from build123d import *

# Parameters (mm, degrees)
F1_R     = 10
F2_DEPTH = 9.2
F3_R     = 37.5
F4_DEPTH = 29.6
F5_R     = 30.5
F6_DEPTH = 25.8
F7_R     = 26.905
F8_DEPTH = 0.35


# Not quite as in the source:
# - a fillet or chamfer that OpenCascade refuses, or shapes differently, is made with other operations: its cross-section is extruded or revolved along the edge and cut away or added


with BuildPart() as f2:
    # F1 (on Top) → F2 (new body)
    with BuildSketch(Plane.XY):
        Circle(F1_R)
    extrude(amount=F2_DEPTH)

    # F3 (on face) → F4 (join)
    with BuildSketch(Plane.XY.offset(9.2)):
        Circle(F3_R)
    extrude(amount=F4_DEPTH)

    # F5 (on face) → F6 (join)
    with BuildSketch(Plane.XY.offset(38.8)):
        Circle(F5_R)
    extrude(amount=F6_DEPTH)

    # F7 (on face) → F8 (cut)
    with BuildSketch(Plane.XY.offset(64.6)):
        Circle(F7_R)
    extrude(amount=-F8_DEPTH, mode=Mode.SUBTRACT)

    # F10: chamfer of 0.5 on 2 edges, made by hand


with BuildPart() as f10_tool2:
    # F10_s3 → F10_t4 (revolve)
    with BuildSketch(Plane.XZ):
        Polygon((27.405, 64.6), (26.905, 64.1), (26.905, 64.6), align=None)
    revolve(axis=Axis((0, 0, 64.6), (0, 0, 1)))

    split(bisect_by=Plane.XY.offset(64.25), keep=Keep.TOP)


with BuildPart() as f2_1:
    add(f2.part)

    # F10_t1: cut F10_tool2
    add(f10_tool2.part, mode=Mode.SUBTRACT)

    # F10_s6 → F10_t7 (revolve, cut)
    with BuildSketch(Plane.XZ):
        Polygon((10, 0.5), (9.5, 0), (10, 0), align=None)
    revolve(axis=Axis((0, 0, 0), (0, 0, 1)), mode=Mode.SUBTRACT)

    # F11 (on Front) → F12 (revolve)
    with BuildSketch(Plane.XZ):
        Polygon((0, 64.25), (0, 74.65), (-19.25, 74.65), (-19.975, 68.05), (-19.975, 64.25), align=None)
    revolve(axis=Axis((0, 0, 44.8884957004), (0, 0, -1)))


solid = f2_1.part
Can you work these out from the model? Positions are in its coordinate system, mm. A direction names the side the tool comes from. Give positions to 0.01 mm unless a question says otherwise; leave off trailing zeros. Order: outer loops, then holes, each group sorted by start corner. A loop starts at its lowest first (then second) coordinate and runs counter-clockwise, first axis right, second up. Notation, with made-up numbers: M -23,8.25 L 12,8.25 A26 cw 12,44.25 Z; hole C -6.75,-2.75 d3. An arc over 180 degrees is marked long. Use one line per item in the form item = value.
Item 1: If we section it at D-D, the plane x = -29: Write out the boundary of the cut face in (y, z).
Values follow:
outline = M -23.77,9.2 L 23.77,9.2 L 23.77,38.8 L 9.45,38.8 L 9.45,64.6 L -9.45,64.6 L -9.45,38.8 L -23.77,38.8 Z
Item 2: If I drill on line 1 along Z through (x, y) = (-23, 5); line 2 along Y through (x, z) = (1, 12); line 3 along Z through (x, y) = (-33, -12.5), over which ranges is the centre line in solid material (lowest first)? Write a range as [from, to].
Values follow:
line_1 = [9.2, 64.25]
line_2 = [-37.49, 37.49]
line_3 = [9.2, 38.8]
Item 3: If we section it at A-A, the plane y = 0: Write out the boundary of the cut face in (x, z) (3 decimals), and give its area (3 significant figures).
Values follow:
outline = M -37.5,9.2 L -10,9.2 L -10,0.5 L -9.5,0 L 9.5,0 L 10,0.5 L 10,9.2 L 37.5,9.2 L 37.5,38.8 L 30.5,38.8 L 30.5,64.6 L 27.405,64.6 L 27.055,64.25 L 19.975,64.25 L 19.975,68.05 L 19.25,74.65 L -19.25,74.65 L -19.975,68.05 L -19.975,64.25 L -27.055,64.25 L -27.405,64.6 L -30.5,64.6 L -30.5,38.8 L -37.5,38.8 Z
area = 4,370 mm^2
Item 4: Thinking about a two-plate mould opening in X: for faces 1 (the cylindrical face through (-24.204, -18.559, 51.519)), 2 (the flat face through (0, 0, 0)), 3 (the flat face through (-10, -18, 64.25)), which applies, pulls with the +X half, pulls with the -X half, needs draft (parallel to the pull), parting line crosses it, or undercut?
Values follow:
face_1 = parting line crosses it
face_2 = needs draft
face_3 = undercut
Item 5: Will these pins go through, and if not, where does the flat tip stop? pin 1 Ø10 at (x, z) = (11.5, 25.5) entering from -Y; pin 2 Ø12 at (x, z) = (11.5, 37.5) entering from +Y; pin 3 Ø12 at (y, z) = (19, 32) entering from +X.
Values follow:
pin_1 = -36.93
pin_2 = 37.09
pin_3 = 35.17
Item 6: For faces 4 (the cylindrical face through (-2.17, -9.76, 4.79)), 5 (the cylindrical face through (-4.88, 37.18, 23.79)), 6 (the cylindrical face through (4.33, -19.5, 66.12)), which set-ups out of +Z, -Z, +X, -X, +Y, -Y let a thin tool reach every point of the face, with its end or its side?
Values follow:
face_4 = -Z
face_5 = +Z, -Z
face_6 = +Z
Item 7: If we section it at C-C, the plane z = 25.5: Write out the boundary of the cut face in (x, y).
Values follow:
outline = C 0,0 d75
